Input: dimensioned drawing with shaded views. Units: mm. Origin: part minimum x, y, z. A direction names the side the tool comes from. Round coordinates to 2 decimals unless told otherwise and drop trailing zeros. Loops run counter-clockwise (first coordinate to the right, second up) from the corner with the lowest first, then second, coordinate; pieces in that order, holes last. Notation, with made-up numbers: (42.25, 48) - (53.25, 48) arc R18 ccw to (53.25, 61) - close; hole circle Ø4 at (-34.75, 19). An arc over 180 degrees is marked (long way). One line per question, with ' | ' between items. Start each with the question number.
Item 1: First-contact query: pin 1 (1.5 mm diameter, centred on x = 243, y = 172.5, fed in from -Z). Flat tip, straight axial feed; report the tip coordinate or a pass-through.
Item 2: Draft query along Z for the marked faces 1, 2 and 3. Return one class per face: pulls with the +Z half, pulls with the -Z half, needs draft (parallel to the pull), parting line crosses it, or undercut.
Item 3: Section A-A, the plane y = 130. Return loops of the section in (x, z).
Item 4: Section B-B, the plane x = 164. Return loops of the section in (y, z).
Item 5: Material intervals for line 1 along Z through (x, y) = (107, 360); line 2 along X through (y, z) = (176, 254), sorted ascending.
Item 6: Section C-C, the plane z = 65. Return loops of the section in (x, y), plus the area to 3 significant figures.
Item 7: Set-up query: the marked faces 4 and 5. Return all of +Z, -Z, +X, -X, +Y, -Y with unobstructed straight access to the full face (end or side cutting, diameter ignored); none if empty.
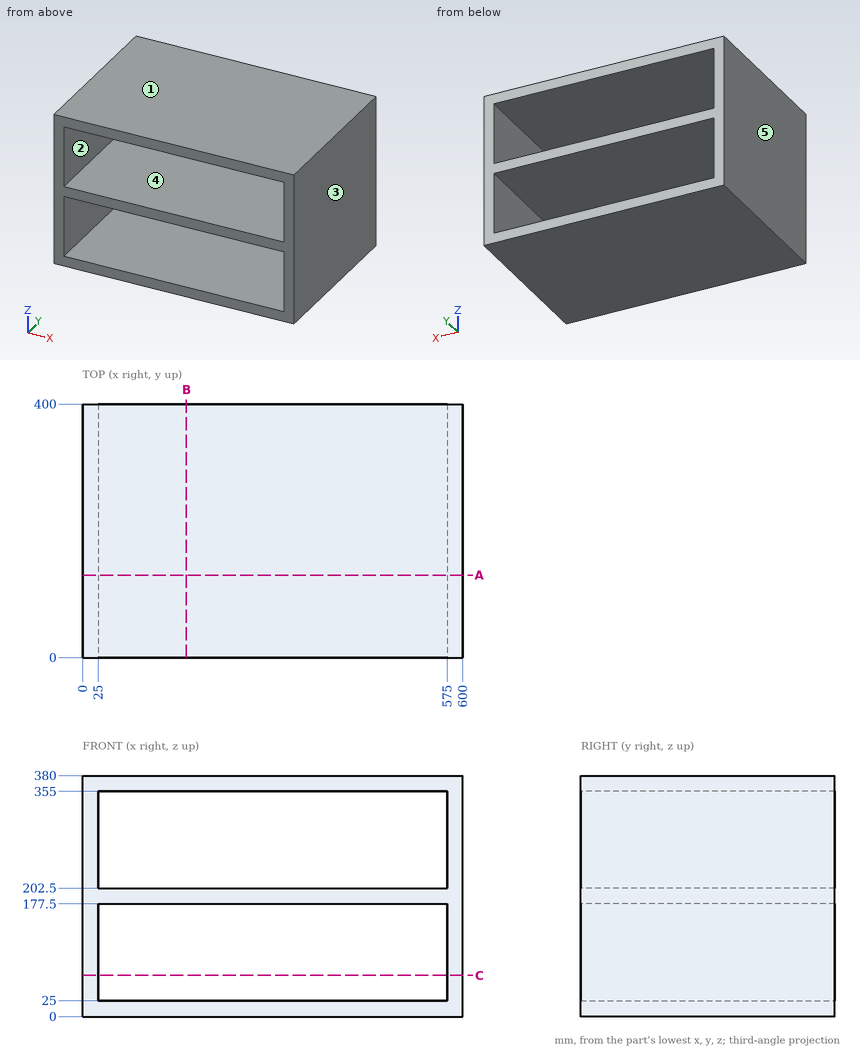
Return value:
1) pin 1: z = 0
2) face 1: pulls with the +Z half | face 2: undercut | face 3: needs draft
3) outline: (0, 0) - (600, 0) - (600, 380) - (0, 380) - close; hole (25, 25) - (575, 25) - (575, 177.5) - (25, 177.5) - close; hole (25, 202.5) - (575, 202.5) - (575, 355) - (25, 355) - close
4) outline: (0, 0) - (400, 0) - (400, 25) - (0, 25) - close; (0, 177.5) - (400, 177.5) - (400, 202.5) - (0, 202.5) - close; (0, 355) - (400, 355) - (400, 380) - (0, 380) - close
5) line 1: 0 to 25, 177.5 to 202.5, 355 to 380 | line 2: 0 to 25, 575 to 600
6) outline: (0, 0) - (25, 0) - (25, 400) - (0, 400) - close; (575, 0) - (600, 0) - (600, 400) - (575, 400) - close | area: 20,000 mm2
7) face 4: +Y, -Y | face 5: +Z, -Z, -X, +Y, -Y
